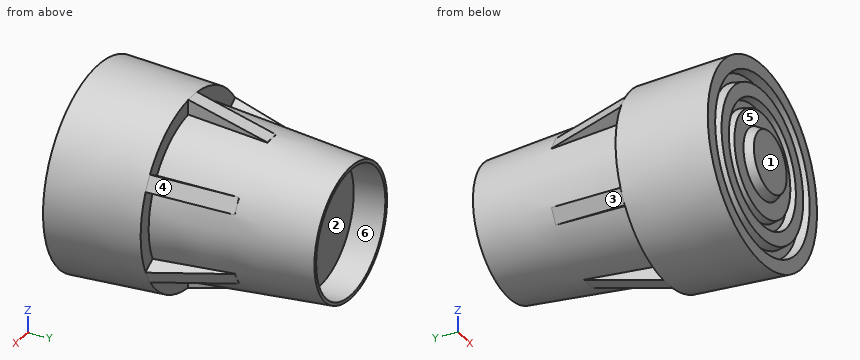
from build123d import *

# Parameters (mm, degrees)
SKETCH1_R           = 21
BOSS_EXTRUDE1_DEPTH = 50
BOSS_EXTRUDE1_DRAFT = 5
SKETCH2_R           = 30
BOSS_EXTRUDE2_DEPTH = 30
BOSS_EXTRUDE2_DRAFT = -3
BOSS_EXTRUDE3_DEPTH = 2.5
CIRPATTERN1_COUNT   = 6
SKETCH4_R           = 27.291330602
SKETCH4_R_2         = 23.594608396
CUT_EXTRUDE1_DEPTH  = 3
CUT_EXTRUDE1_DRAFT  = -10
SKETCH5_R           = 19.382333363
SKETCH5_R_2         = 16.172751495
CUT_EXTRUDE2_DEPTH  = 2.5
CUT_EXTRUDE2_DRAFT  = -10
SKETCH6_R           = 10.925848264
BOSS_EXTRUDE4_DEPTH = 2.5
BOSS_EXTRUDE4_TAPER = 30
SKETCH7_R           = 20
CUT_EXTRUDE3_DEPTH  = 10


with BuildPart() as part:
    # Sketch1 → Boss-Extrude1 (with draft: the straight prism first)
    with BuildSketch(Plane(origin=(0, 0, 0), x_dir=(1, 0, 0), z_dir=(0, 1, 0))):
        Circle(SKETCH1_R)
    extrude(amount=-BOSS_EXTRUDE1_DEPTH)
    # Boss-Extrude1: the draft: its side faces are tilted about the plane it starts from
    boss_extrude1_sides = [part.faces().sort_by_distance(p)[0] for p in [
        (-21, -25, 0),
    ]]
    draft(boss_extrude1_sides, Plane(origin=(0, 0, 0), x_dir=(1, 0, 0), z_dir=(0, 1, 0)), BOSS_EXTRUDE1_DRAFT)


with BuildPart() as boss_extrude2_tool:
    # Sketch2 → Boss-Extrude2 (with draft: the straight prism first)
    with BuildSketch(Plane.XZ.offset(50)):
        Circle(SKETCH2_R)
    extrude(amount=BOSS_EXTRUDE2_DEPTH)
    # Boss-Extrude2: the draft: its side faces are tilted about the plane it starts from
    boss_extrude2_sides = [boss_extrude2_tool.faces().sort_by_distance(p)[0] for p in [
        (-30, -65, 0),
    ]]
    draft(boss_extrude2_sides, Plane.XZ.offset(50), BOSS_EXTRUDE2_DRAFT)


with BuildPart() as part_1:
    add(part.part)

    # Boss-Extrude2: add boss_extrude2_tool
    add(boss_extrude2_tool.part)

    # Sketch3 → Boss-Extrude3 (add, symmetric)
    with BuildSketch(Plane(origin=(0, 0, 0), x_dir=(0, 0, -1), z_dir=(1, 0, 0))):
        Polygon((-25.374433176, -50), (-30, -50), (-23.187216588, -25), (-20.280513913, -25), (-22.467730501, -50), align=None)
    boss_extrude3 = extrude(amount=BOSS_EXTRUDE3_DEPTH, both=True)

    # CirPattern1: Boss-Extrude3 ×6 about axis
    cirpattern1_axis = Axis((0, 0, 0), (0, 1, 0))
    for i in range(1, CIRPATTERN1_COUNT):
        add(boss_extrude3.rotate(cirpattern1_axis, i * 360 / CIRPATTERN1_COUNT))


with BuildPart() as cut_extrude1_tool:
    # Sketch4 → Cut-Extrude1 (with draft: the straight prism first)
    with BuildSketch(Plane.XZ.offset(80)):
        Circle(SKETCH4_R)
        Circle(SKETCH4_R_2, mode=Mode.SUBTRACT)
    extrude(amount=-CUT_EXTRUDE1_DEPTH)
    # Cut-Extrude1: the draft: its side faces are tilted about the plane it starts from
    cut_extrude1_sides = [cut_extrude1_tool.faces().sort_by_distance(p)[0] for p in [
        (-27.291330602, -78.5, 0),
        (-23.594608396, -78.5, 0),
    ]]
    draft(cut_extrude1_sides, Plane.XZ.offset(80), CUT_EXTRUDE1_DRAFT)


with BuildPart() as part_2:
    add(part_1.part)

    # Cut-Extrude1: cut by cut_extrude1_tool
    add(cut_extrude1_tool.part, mode=Mode.SUBTRACT)


with BuildPart() as cut_extrude2_tool:
    # Sketch5 → Cut-Extrude2 (with draft: the straight prism first)
    with BuildSketch(Plane.XZ.offset(80)):
        Circle(SKETCH5_R)
        Circle(SKETCH5_R_2, mode=Mode.SUBTRACT)
    extrude(amount=-CUT_EXTRUDE2_DEPTH)
    # Cut-Extrude2: the draft: its side faces are tilted about the plane it starts from
    cut_extrude2_sides = [cut_extrude2_tool.faces().sort_by_distance(p)[0] for p in [
        (-19.382333363, -78.75, 0),
        (-16.172751495, -78.75, 0),
    ]]
    draft(cut_extrude2_sides, Plane.XZ.offset(80), CUT_EXTRUDE2_DRAFT)


with BuildPart() as part_3:
    add(part_2.part)

    # Cut-Extrude2: cut by cut_extrude2_tool
    add(cut_extrude2_tool.part, mode=Mode.SUBTRACT)

    # Sketch6 → Boss-Extrude4 (add)
    with BuildSketch(Plane.XZ.offset(80)):
        Circle(SKETCH6_R)
    extrude(amount=BOSS_EXTRUDE4_DEPTH, taper=BOSS_EXTRUDE4_TAPER)

    # Sketch7 → Cut-Extrude3 (cut)
    with BuildSketch(Plane(origin=(0, 0, 0), x_dir=(1, 0, 0), z_dir=(0, 1, 0))):
        with Locations(Location((0, 0, 0), (0, 0, 270))):
            Circle(SKETCH7_R)
    extrude(amount=-CUT_EXTRUDE3_DEPTH, mode=Mode.SUBTRACT)


solid = part_3.part
Design review of the part built by this model. Coordinates are the model's own, in mm. Face numbers are marked on the shaded views. A direction names the side the tool comes from. Give positions to 0.01 mm unless a question says otherwise; leave off trailing zeros. Loops run counter-clockwise (first coordinate to the right, second up) from the corner with the lowest first, then second, coordinate; pieces in that order, holes last. Notation, with made-up numbers: M 60,83 L 64,83 A15 ccw 64,97 Z; hole C 28.5,63 d11. An arc over 180 degrees is marked long. Answer as a JSON object with one key per item and string values.
Item 1: We need section A-A (y = -38.5). State the section outline as (x, z) points, and give its area (3 significant figures).
Output values:
{"outline": "M -24.52,-11.27 L -22.02,-15.6 L -19.74,-14.28 A24.37 ccw -2.5,-24.24 L -2.5,-26.87 L 2.5,-26.87 L 2.5,-24.24 A24.37 ccw 19.74,-14.28 L 22.02,-15.6 L 24.52,-11.27 L 22.24,-9.95 A24.37 ccw 22.24,9.95 L 24.52,11.27 L 22.02,15.6 L 19.74,14.28 A24.37 ccw 2.5,24.24 L 2.5,26.87 L -2.5,26.87 L -2.5,24.24 A24.37 ccw -19.74,14.28 L -22.02,15.6 L -24.52,11.27 L -22.24,9.95 A24.37 ccw -22.24,-9.95 Z", "area": "1,940 mm2"}
Item 2: Machinability: for the marked faces 5 and 6, which of the approach directions +Z, -Z, +X, -X, +Y, -Y give a long, thin tool a straight path to every point of the face, cutting with its end or side? Answer none if there is none.
Output values:
{"face 5": "-Y", "face 6": "+Y"}
Item 3: We need section B-B (y = -63.5). State the section outline as (x, z) points, and give its area (3 significant figures).
Output values:
{"outline": "C 0,0 d61.42", "area": "2,960 mm2"}
Item 4: For P1, Ø5, axis at x = 6.5, z = 12, coming from the +Y side; P2, Ø3.5, axis at y = -36, z = -26.5, coming from the -X side; P3, Ø1.5, axis at x = -11, z = 18.5, coming from the -Y side, all flat-tipped, find the tip position at first contact; note any pin that passes through.
Output values:
{"P1": "stops at y = -10", "P2": "stops at x = -2.5", "P3": "stops at y = -80"}
Item 5: We need section C-C (y = -24). State the section outline as (x, z) points, and give its area (3 significant figures).
Output values:
{"outline": "C 0,0 d46.2", "area": "1,680 mm2"}
Item 6: Mouldability with a two-part tool opening along Z and no side actions: class the marked faces 1, 2, 3 and 4 as pulls with the +Z half, pulls with the -Z half, needs draft (parallel to the pull), parting line crosses it, or undercut.
Output values:
{"face 1": "needs draft", "face 2": "undercut", "face 3": "pulls with the -Z half", "face 4": "pulls with the +Z half"}
Item 7: Wall thickness on line 1 along X through (y, z) = (-4, 0); line 2 along Y through (x, z) = (13.5, 14.5); line 3 along X through (y, z) = (-5.75, 0): over which ranges is each line inside the solid? List them lowest first.
Output values:
{"line 1": "x = -21.35 to -20, 20 to 21.35", "line 2": "y = -80 to -10", "line 3": "x = -21.5 to -20, 20 to 21.5"}
